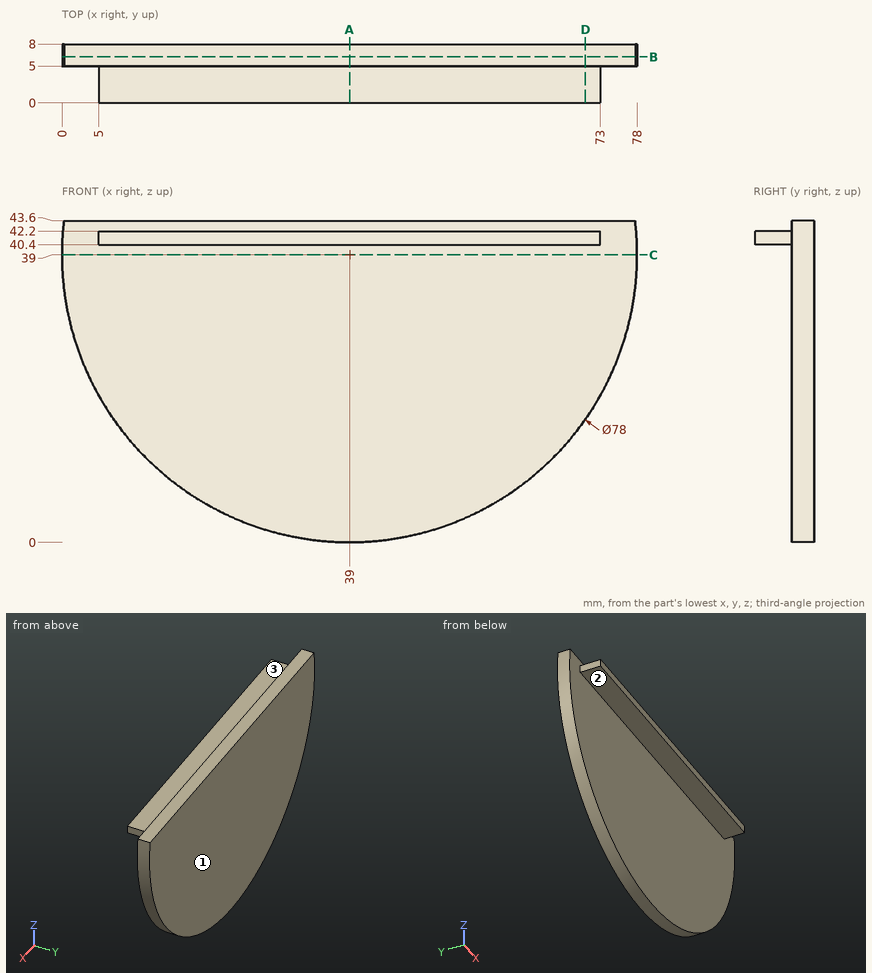
Geometry check sheet. Reference: drawing and pictorial views, mm from the part's lowest x, y, z. A direction names the side the tool comes from. Round coordinates to 2 decimals unless told otherwise and drop trailing zeros. Write each loop counter-clockwise with the first axis right and the second up, starting at its lowest first coordinate (ties: lowest second). Pieces come first, ordered by that corner, then holes. Notation, with made-up numbers: (-23, -33) -> (-5, -33) arc R27 ccw to (-5, -5) -> close; hole circle Ø10 at (37.25, 5.5). An arc over 180 degrees is marked (long way). Put each result on its own line as item: value.
1) Cross-section at A-A, the plane x = 39. Enter the section's corners in (y, z), plus the area to 3 significant figures.
Recorded:
outline: (0, 40.4) -> (5, 40.4) -> (5, 0) -> (8, 0) -> (8, 43.6) -> (5, 43.6) -> (5, 42.2) -> (0, 42.2) -> close
area: 140 mm2
2) Access from +Z, -Z, +X, -X, +Y, -Y to the whole of each face (thin tool, end or side, straight path). Record for the marked faces 1, 2 and 3.
Recorded:
face 1: +Z, -Z, +X, -X, +Y
face 2: -Z, +X, -X, -Y
face 3: +Z, +X, -X, -Y
3) Cross-section at D-D, the plane x = 71. Enter the section's corners in (y, z), plus the area to 3 significant figures.
Recorded:
outline: (0, 40.4) -> (5, 40.4) -> (5, 16.71) -> (8, 16.71) -> (8, 43.6) -> (5, 43.6) -> (5, 42.2) -> (0, 42.2) -> close
area: 89.7 mm2
4) Thickness scan on probe 1 along Y at (x, z) = (71, 23.5); probe 2 along Z at (x, y) = (38, 7.25); probe 3 along Z at (x, y) = (20, 4.25). Record the ranges inside material, lowest first. Write a range as from..to.
Recorded:
probe 1: y = 5..8
probe 2: z = 0.01..43.6
probe 3: z = 40.4..42.2
5) Depth check by flat-ended pin: P1, Ø1.5, axis at x = 8, y = 4, coming from the +Z side; P2, Ø8, axis at x = 39, z = 35.5, coming from the -Y side; P3, Ø2, axis at y = 3.5, z = 41.5, coming from the -X side. Enter the tip coordinate at first touch or a pass-through.
Recorded:
P1: stops at z = 42.2
P2: stops at y = 5
P3: stops at x = 5
6) Cross-section at C-C, the plane z = 39. Enter the section's corners in (x, y), plus the area to 3 significant figures.
Recorded:
outline: (0, 5) -> (78, 5) -> (78, 8) -> (0, 8) -> close
area: 234 mm2
7) Cross-section at B-B, the plane y = 6.25. Enter the section's corners in (x, z).
Recorded:
outline: (0.27, 43.6) arc R39 ccw (long way) to (77.73, 43.6) -> close
